```python
from build123d import *

# Parameters (mm, degrees)
F2_R     = 1.33
F3_DEPTH = 12.5


with BuildPart() as f1:
    # F0 (on Front) → F1 (revolve)
    with BuildSketch(Plane.XZ):
        Polygon((7, -1.05), (7, 0), (1.5, 0), (1.5, 2.5), (0, 2.5), (0, 0), (0, -2.1), (6.2, -2.1), (6.2, -2.5), (7, -2.5), align=None)
    revolve(axis=Axis((0, 0, 1.25), (0, 0, 1)))

    # F2 (on Front) → F3 (cut, symmetric)
    with BuildSketch(Plane.XZ):
        with Locations((0, 2.523782)):
            Circle(F2_R)
    extrude(amount=F3_DEPTH, both=True, mode=Mode.SUBTRACT)


solid = f1.part
```
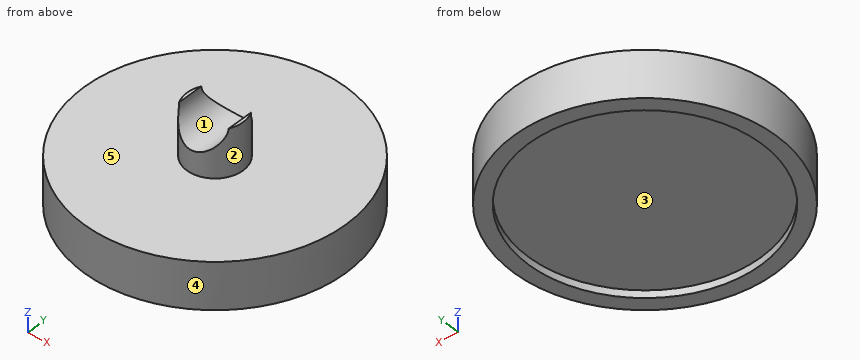
The model under review builds one solid part; all positions refer to its coordinate system, in mm. Face numbers are marked on the shaded views. A direction names the side the tool comes from. Round coordinates to 2 decimals unless told otherwise and drop trailing zeros. Write each loop counter-clockwise with the first axis right and the second up, starting at its lowest first coordinate (ties: lowest second). Pieces come first, ordered by that corner, then holes. Notation, with made-up numbers: M 32.25,3 L 72.25,3 A27 cw 72.25,34 Z; hole C -9.75,69.25 d1. An arc over 180 degrees is marked long. Use CSV: the item, a comma, the result in double quotes. Start each with the question number.
(1) Tool access review of the marked faces 1 and 2: name each direction out of +Z, -Z, +X, -X, +Y, -Y from which nothing blocks a thin tool from reaching the whole face with its end or side.
(2) We need section D-D, the plane z = -0.4. State the section outline as (x, y) points, then the cut area to 3 significant figures.
(3) The part is to be moulded in two halves that separate along X. For the marked faces 3, 4 and 5, say which applies: +X half, -X half, draft (parallel to the pull), parting line (faces both ways), or undercut.
(4) We need section C-C, the plane z = 2.15. State the section outline as (x, y) points.
(5) For line 1 along Y through (x, z) = (0, -2.2); line 2 along Z through (x, y) = (-5.75, 3.5); line 3 along Z through (x, y) = (5.5, 0.5), list the stretches that pass through material, from the lowest coordinate up.
(6) We need section B-B, the plane y = 0. State the section outline as (x, z) points.
(7) Clearance check with flat-ended pins moving along their axes: P1, Ø2, axis at y = 3, z = 0, coming from the -X side; P2, Ø6, axis at x = 0, y = 2, coming from the -Z side. State where each tip first meets the part, or that it passes through.
(8) We need section A-A, the plane x = 0. State the section outline as (y, z) points, then the cut area to 3 significant figures.
Findings:
1,face 1,"+Z, +Y, -Y"
1,face 2,"+Z"
2,outline,"C 0,0 d14"
2,area,"154 mm^2"
3,face 3,"undercut"
3,face 4,"parting line"
3,face 5,"draft"
4,outline,"M -1.28,-0.79 L -1.28,0.79 A1.5 ccw Z; M 1.28,-0.79 A1.5 ccw 1.28,0.79 Z"
5,line 1,"-7 to -6.2, 6.2 to 7"
5,line 2,"-2.5 to 0"
5,line 3,"-2.1 to 0"
6,outline,"M -7,-2.5 L -6.2,-2.5 L -6.2,-2.1 L 6.2,-2.1 L 6.2,-2.5 L 7,-2.5 L 7,0 L 1.5,0 L 1.5,2.5 L 1.33,2.5 A1.33 cw -1.33,2.5 L -1.5,2.5 L -1.5,0 L -7,0 Z"
7,P1,"x = -6.71"
7,P2,"z = -2.1"
8,outline,"M -7,-2.5 L -6.2,-2.5 L -6.2,-2.1 L 6.2,-2.1 L 6.2,-2.5 L 7,-2.5 L 7,0 L 1.5,0 L 1.5,1.19 L -1.5,1.19 L -1.5,0 L -7,0 Z"
8,area,"33.6 mm^2"
